```python
from build123d import *

# Parameters (mm, degrees)
PAD_DEPTH    = 3
SKETCH001_W  = 16.2
SKETCH001_H  = 1.2
POCKET_DEPTH = 1.5
PAD001_DEPTH = 1


with BuildPart() as part:
    # Sketch → Pad (new body)
    with BuildSketch(Plane.XY):
        with BuildLine():
            Line((6.1, 33.346624), (-6.1, 33.346624))
            Line((-6.1, 33.346624), (-6.1, 27.946624))
            Line((-6.1, 27.946624), (-8.1, 27.946624))
            Line((-8.1, 27.946624), (-8.1, 25.546624))
            ThreePointArc((8.1, 25.546624), (0, 26.8), (-8.1, 25.546624))
            Line((8.1, 27.946624), (8.1, 25.546624))
            Line((6.1, 27.946624), (8.1, 27.946624))
            Line((6.1, 33.346624), (6.1, 27.946624))
        make_face()
    extrude(amount=PAD_DEPTH)

    # Sketch001 (on DatumPlane) → Pocket (cut)
    with BuildSketch(Plane(origin=(2.7, 25.546624, 1), x_dir=(1, 0, 0), z_dir=(0, -1, 0))):
        with Locations((-2.7, 0.5)):
            Rectangle(SKETCH001_W, SKETCH001_H)
    extrude(amount=-POCKET_DEPTH, mode=Mode.SUBTRACT)

    # Sketch002 (on Face5 of Pocket) → Pad001 (join)
    with BuildSketch(Plane.XY.offset(3)):
        with BuildLine():
            ThreePointArc((0.5, 27.8), (0, 28.3), (-0.5, 27.8))
            Line((-0.5, 27.8), (-0.5, 26.795335))
            ThreePointArc((0.5, 26.795335), (0, 26.8), (-0.5, 26.795335))
            Line((0.5, 27.8), (0.5, 26.795335))
        make_face()
    extrude(amount=PAD001_DEPTH)


solid = part.part
```
Design review of the part built by this model. Coordinates are the model's own, in mm. A direction names the side the tool comes from. Coordinates: 2 decimals unless noted, no trailing zeros. Loops run counter-clockwise (first coordinate to the right, second up) from the corner with the lowest first, then second, coordinate; pieces in that order, holes last. Notation, with made-up numbers: (-7, 78) - (6, 78) arc R21 ccw to (6, 97) - close; hole circle Ø4 at (69.25, 41). An arc over 180 degrees is marked (long way). Use CSV: the item, a comma, the result in double quotes. Start each with the question number.
1) Consider section B-B on z = 2.5. Write out the cut boundary in (x, y), then the cut area to 3 significant figures.
2) Consider section D-D on y = 29.75. Write out the cut boundary in (x, z).
3) The part is to be moulded in two halves that separate along X. For faces 1 (the cylindrical face through (0.1, 26.8, 2.5)), 2 (the flat face through (-8.1, 27.3, 1.5)), say which applies: +X half, -X half, draft (parallel to the pull), parting line (faces both ways), or undercut.
4) Consider section C-C on z = 1.8. Write out the cut boundary in (x, y), then the cut area to 3 significant figures.
5) Tool access review of faces 3 (the flat face through (7, 27.947, 1)), 4 (the cylindrical face through (0, 28.3, 3.5)), 5 (the flat face through (-0.5, 27.3, 3.5)), 6 (the flat face through (-0.1, 27.047, 1.5)), 7 (the flat face through (-7, 27.947, 1)): name each direction out of +Z, -Z, +X, -X, +Y, -Y from which nothing blocks a thin tool from reaching the whole face with its end or side.
6) For pin 1 Ø0.5 at (y, z) = (27.5, 3.5) entering from -X; pin 2 Ø3 at (x, y) = (-3.5, 32.5) entering from +Z; pin 3 Ø2 at (x, z) = (-7.5, 1.5) entering from +Y, all flat-tipped, find the tip position at first contact; note any pin that passes through.
7) Wall thickness on L1, parallel to X at y = 29.25, z = 2.65; L2, parallel to Z at x = 3, y = 31.25; L3, parallel to Z at x = -6.25, y = 26.5: over which ranges is each line inside the solid? List them lowest first. Write a range as from..to.
8) Consider section A-A on x = 0. Write out the cut boundary in (y, z), then the cut area to 3 significant figures.
Geometry says:
1,outline,"(-8.1, 25.55) arc R26.8 cw to (8.1, 25.55) - (8.1, 27.95) - (6.1, 27.95) - (6.1, 33.35) - (-6.1, 33.35) - (-6.1, 27.95) - (-8.1, 27.95) - close"
1,area,"91.2 mm^2"
2,outline,"(-6.1, 0) - (6.1, 0) - (6.1, 3) - (-6.1, 3) - close"
3,face 1,"undercut"
3,face 2,"-X half"
4,outline,"(-8.1, 27.05) - (8.1, 27.05) - (8.1, 27.95) - (6.1, 27.95) - (6.1, 33.35) - (-6.1, 33.35) - (-6.1, 27.95) - (-8.1, 27.95) - close"
4,area,"80.5 mm^2"
5,face 3,"+Z, -Z, +X, +Y"
5,face 4,"+Z, +Y"
5,face 5,"+Z, -X, +Y, -Y"
5,face 6,"+X, -X, -Y"
5,face 7,"+Z, -Z, -X, +Y"
6,pin 1,"x = -0.5"
6,pin 2,"z = 3"
6,pin 3,"y = 27.95"
7,L1,"-6.1..6.1"
7,L2,"0..3"
7,L3,"0..0.9, 2.1..3"
8,outline,"(26.8, 0) - (33.35, 0) - (33.35, 3) - (28.3, 3) - (28.3, 4) - (26.8, 4) - (26.8, 2.1) - (27.05, 2.1) - (27.05, 0.9) - (26.8, 0.9) - close"
8,area,"20.8 mm^2"
